Could you check a few things on this model? Use its own coordinates, in mm. A direction names the side the tool comes from. Give positions to 0.01 mm unless a question says otherwise; leave off trailing zeros. Write each loop counter-clockwise with the first axis right and the second up, starting at its lowest first coordinate (ties: lowest second). Pieces come first, ordered by that corner, then holes. Notation, with made-up numbers: (-3.5, -31) - (25.5, -31) arc R32 ccw to (25.5, -3) - close; hole circle Ø1 at (8.25, 2). An arc over 180 degrees is marked (long way). Write item = value, one per line.
from build123d import *

# Parameters (mm, degrees)
EXTRUDE_DEPTH        = 1
SKETCH_W             = 18
SKETCH_H             = 18
PAD_DEPTH            = 8
POCKET_DEPTH         = 18.001
POCKET001_DEPTH      = 9.001
POCKET001_DEPTH_BACK = 9.001
FILLET_R             = 2
THICKNESS_T          = -1


with BuildPart() as extrude_body:
    # Sketch003 → Extrude (new body)
    with BuildSketch(Plane.XY):
        with BuildLine():
            add(Edge.make_bspline(
                [(0, 0.5656), (0.587711, 1.0828)],
                knots=[0, 0, 1, 1], degree=1))
            add(Edge.make_bspline(
                [(0.587711, 1.0828), (0.909016, 1.35583), (1.22484, 1.07789), (1.54067, 0.799956), (1.23042, 0.517199)],
                knots=[0, 0, 0, 0.333333, 0.666667, 1, 1, 1], degree=2))
            add(Edge.make_bspline(
                [(1.23042, 0.517199), (0.642707, 0)],
                knots=[0, 0, 1, 1], degree=1))
            add(Edge.make_bspline(
                [(0.642707, 0), (1.23042, -0.517202)],
                knots=[0, 0, 1, 1], degree=1))
            add(Edge.make_bspline(
                [(1.23042, -0.517202), (1.54067, -0.799959), (1.22484, -1.0779), (0.909016, -1.35583), (0.587711, -1.0828)],
                knots=[0, 0, 0, 0.333333, 0.666667, 1, 1, 1], degree=2))
            add(Edge.make_bspline(
                [(0.587711, -1.0828), (0, -0.5656)],
                knots=[0, 0, 1, 1], degree=1))
            add(Edge.make_bspline(
                [(0, -0.5656), (-0.587708, -1.0828)],
                knots=[0, 0, 1, 1], degree=1))
            add(Edge.make_bspline(
                [(-0.587708, -1.0828), (-0.909014, -1.3559), (-1.22488, -1.07793), (-1.54074, -0.79996), (-1.23042, -0.517202)],
                knots=[0, 0, 0, 0.333333, 0.666667, 1, 1, 1], degree=2))
            add(Edge.make_bspline(
                [(-1.23042, -0.517202), (-0.642707, 0)],
                knots=[0, 0, 1, 1], degree=1))
            add(Edge.make_bspline(
                [(-0.642707, 0), (-1.23042, 0.517199)],
                knots=[0, 0, 1, 1], degree=1))
            add(Edge.make_bspline(
                [(-1.23042, 0.517199), (-1.54074, 0.799958), (-1.22488, 1.07793), (-0.909014, 1.3559), (-0.587708, 1.0828)],
                knots=[0, 0, 0, 0.333333, 0.666667, 1, 1, 1], degree=2))
            add(Edge.make_bspline(
                [(-0.587708, 1.0828), (0, 0.5656)],
                knots=[0, 0, 1, 1], degree=1))
        make_face()
        with BuildLine():
            Line((-0.613575, -3), (-2.35447, -3))
            add(Edge.make_bspline(
                [(-2.35447, -3), (-2.85946, -3), (-3.49148, -2.7568), (-3.83261, -2.4312)],
                knots=[0, 0, 0, 0, 1, 1, 1, 1], degree=3))
            add(Edge.make_bspline(
                [(-3.83261, -2.4312), (-5.57096, -0.772401)],
                knots=[0, 0, 1, 1], degree=1))
            add(Edge.make_bspline(
                [(-5.57096, -0.772401), (-6.02186, -0.3424), (-6.02208, 0.341998), (-5.57096, 0.772398)],
                knots=[0, 0, 0, 0, 1, 1, 1, 1], degree=3))
            add(Edge.make_bspline(
                [(-5.57096, 0.772398), (-3.83238, 2.4312)],
                knots=[0, 0, 1, 1], degree=1))
            add(Edge.make_bspline(
                [(-3.83238, 2.4312), (-3.49216, 2.756), (-2.85809, 3), (-2.35447, 3)],
                knots=[0, 0, 0, 0, 1, 1, 1, 1], degree=3))
            Line((-2.35447, 3), (-0.619992, 3))
            Line((-0.619992, 3), (-0.619992, 2.2))
            Line((-0.619992, 2.2), (-2.35447, 2.2))
            add(Edge.make_bspline(
                [(-2.35447, 2.2), (-2.60446, 2.2), (-2.99604, 2.0494), (-3.16422, 1.8888)],
                knots=[0, 0, 0, 0, 1, 1, 1, 1], degree=3))
            add(Edge.make_bspline(
                [(-3.16422, 1.8888), (-4.9028, 0.230198)],
                knots=[0, 0, 1, 1], degree=1))
            add(Edge.make_bspline(
                [(-4.9028, 0.230198), (-5.03257, 0.106198), (-5.03234, -0.106201), (-4.9028, -0.230201)],
                knots=[0, 0, 0, 0, 1, 1, 1, 1], degree=3))
            add(Edge.make_bspline(
                [(-4.9028, -0.230201), (-3.16422, -1.8888)],
                knots=[0, 0, 1, 1], degree=1))
            add(Edge.make_bspline(
                [(-3.16422, -1.8888), (-2.99536, -2.05), (-2.6056, -2.2), (-2.35447, -2.198788)],
                knots=[0, 0, 0, 0, 1, 1, 1, 1], degree=3))
            Line((-2.35447, -2.198788), (-0.613575, -2.198788))
            Line((-0.613575, -2.198788), (-0.613575, -3))
        make_face()
        with BuildLine():
            add(Edge.make_bspline(
                [(2.95332, 3), (4.09261, 3.001), (4.09078, 1.9984)],
                knots=[0, 0, 0, 1, 1, 1], degree=2))
            add(Edge.make_bspline(
                [(4.09078, 1.9984), (4.09078, -1.9984)],
                knots=[0, 0, 1, 1], degree=1))
            add(Edge.make_bspline(
                [(4.09078, -1.9984), (4.09169, -3), (2.95354, -3)],
                knots=[0, 0, 0, 1, 1, 1], degree=2))
            Line((2.95354, -3), (0.585592, -3))
            Line((0.585592, -3), (0.585592, -2.20349))
            Line((0.585592, -2.20349), (2.95354, -2.20349))
            add(Edge.make_bspline(
                [(2.95354, -2.20349), (3.07945, -2.2), (3.18172, -2.1102), (3.18172, -1.9984)],
                knots=[0, 0, 0, 0, 1, 1, 1, 1], degree=3))
            add(Edge.make_bspline(
                [(3.18172, -1.9984), (3.18172, 1.9984)],
                knots=[0, 0, 1, 1], degree=1))
            add(Edge.make_bspline(
                [(3.18172, 1.9984), (3.18172, 2.1104), (3.08036, 2.2), (2.95354, 2.2)],
                knots=[0, 0, 0, 0, 1, 1, 1, 1], degree=3))
            Line((2.95354, 2.2), (0.586243, 2.2))
            Line((0.586243, 2.2), (0.586243, 3))
            Line((0.586243, 3), (2.95332, 3))
        make_face()
    extrude(amount=EXTRUDE_DEPTH)


with BuildPart() as extrude_body_1:
    # Extrude placement: moved
    add(extrude_body.part.moved(Location((1, 0, 7))))


with BuildPart() as cut:
    # Sketch → Pad (new body)
    with BuildSketch(Plane.XY):
        Rectangle(SKETCH_W, SKETCH_H)
    extrude(amount=PAD_DEPTH)

    # Sketch001 (on Face1 of Pad) → Pocket (cut, through all)
    with BuildSketch(Plane.XZ.offset(9)):
        Polygon((-9, 8), (-9, 0), (-7, 8), align=None)
        Polygon((9, 8), (9, 0), (7, 8), align=None)
    extrude(amount=-POCKET_DEPTH, mode=Mode.SUBTRACT)

    # Sketch002 → Pocket001 (cut, two sides)
    with BuildSketch(Plane.YZ) as pocket001_sk:
        Polygon((-9, 8), (-7, 8), (-9, 0), align=None)
        Polygon((9, 8), (7, 8), (9, 0), align=None)
    extrude(amount=-POCKET001_DEPTH, mode=Mode.SUBTRACT)
    extrude(pocket001_sk.sketch, amount=POCKET001_DEPTH_BACK, mode=Mode.SUBTRACT)

    # Fillet
    fillet_edges = [cut.edges().sort_by_distance(p)[0] for p in [
        (-8, 8, 4),
        (-8, -8, 4),
        (8, -8, 4),
        (8, 8, 4),
    ]]
    fillet(fillet_edges, radius=FILLET_R)

    # Thickness
    thickness_openings = [cut.faces().sort_by_distance(p)[0] for p in [
        (0, 0, 0),
    ]]
    offset(amount=THICKNESS_T, openings=thickness_openings, kind=Kind.INTERSECTION)

    # Cut: cut Extrude body
    add(extrude_body_1.part, mode=Mode.SUBTRACT)


solid = cut.part
1. Which directions (+Z, -Z, +X, -X, +Y, -Y) give clear straight access to the entire face, cutting with the end or side of a thin tool? Please do faces 1 (the face through (6.8, -6.78, 3.59)), 2 (the face through (-0.5, -2.199, 7.5)), 3 (the face through (0, 8, 4)).
Filled sheet:
face_1 = -Z
face_2 = +Z, -Z
face_3 = +Z, +X, -X, +Y
2. I need wall thicknesses on line 1 (Y direction, x = -1.25, z = 7.5) (3 decimals); line 2 (Z direction, x = 0.25, y = 4); line 3 (Y direction, x = -3, z = 6.5) (3 decimals). Which ranges of each line are inside material? Lowest first, please.
Filled sheet:
line_1 = -7.125 to -3, -2.199 to 2.2, 3 to 7.125
line_2 = 7 to 8
line_3 = -7.375 to -6.344, 6.344 to 7.375
3. For pin 1 (1.1 mm diameter, centred on x = 2.5, z = 7.5, fed in from +Y); pin 2 (1.5 mm diameter, centred on x = -5, z = 2.5, fed in from -Y); pin 3 (3.5 mm diameter, centred on x = -0.5, y = 1.5, fed in from -Z), each with a flat end and sliding along its axis, tell me the tip position at first contact or that it passes through.
Filled sheet:
pin_1 = 7.26
pin_2 = -8.56
pin_3 = 7
4. If we section it at A-A, the plane x = -1: Please give me the cut outline in (y, z), and give its area (3 significant figures).
Filled sheet:
outline = (-9, 0) - (-7.97, 0) - (-6.22, 7) - (-3, 7) - (-3, 8) - (-7, 8) - close; (-2.2, 7) - (2.2, 7) - (2.2, 8) - (-2.2, 8) - close; (3, 7) - (6.22, 7) - (7.97, 0) - (9, 0) - (7, 8) - (3, 8) - close
area = 27.1 mm2
5. If we section it at B-B, the plane y = -3.25: Please give me the cut outline in (x, z).
Filled sheet:
outline = (-9, 0) - (-7.97, 0) - (-6.22, 7) - (6.22, 7) - (7.97, 0) - (9, 0) - (7, 8) - (-7, 8) - close
6. If we section it at C-C, the plane z = 7.75: Count the separate pieces of the cut face and the enclosed holes in it, and give its area (3 significant figures).
Filled sheet:
separate_pieces = 1
enclosed_holes = 3
area = 172 mm2
7. Thinking about a two-plate mould opening in Y: for faces 4 (the face through (0, -8, 4)), 5 (the face through (-8, 0, 4)), 6 (the face through (2.8, -2.203, 7.5)), 7 (the face through (7.395, 7.425, 4.112)), which applies, pulls with the +Y half, pulls with the -Y half, needs draft (parallel to the pull), parting line crosses it, or undercut?
Filled sheet:
face_4 = pulls with the -Y half
face_5 = needs draft
face_6 = undercut
face_7 = pulls with the +Y half
